```python
from build123d import *

# Parameters (mm, degrees)
IZIM2_W                     = 79
IZIM2_H                     = 44
IZIM2_R                     = 6.5
IZIM2_R_2                   = 1
IZIM2_R_3                   = 13
Y_KSEKLIK_EKSTR_ZYON1_DEPTH = 4
IZIM3_R                     = 15
IZIM3_R_2                   = 13
Y_KSEKLIK_EKSTR_ZYON2_DEPTH = 4


with BuildPart() as part:
    # Çizim2 → Yükseklik-Ekstrüzyon1 (new body)
    with BuildSketch(Plane(origin=(0, 0, 0), x_dir=(1, 0, 0), z_dir=(0, 1, 0))):
        with Locations((-17.5, 0)):
            Rectangle(IZIM2_W, IZIM2_H)
        with Locations(Location((0, 0, 0), (0, 0, 270))):
            Circle(IZIM2_R, mode=Mode.SUBTRACT)
        with Locations(Location((0, 12.5, 0), (0, 0, 270))):
            Circle(IZIM2_R_2, mode=Mode.SUBTRACT)
        with Locations(Location((0, -12.5, 0), (0, 0, 270))):
            Circle(IZIM2_R_2, mode=Mode.SUBTRACT)
        with Locations(Location((-35, 0, 0), (0, 0, 270))):
            Circle(IZIM2_R_3, mode=Mode.SUBTRACT)
    extrude(amount=Y_KSEKLIK_EKSTR_ZYON1_DEPTH)

    # Çizim3 → Yükseklik-Ekstrüzyon2 (add)
    with BuildSketch(Plane(origin=(0, 4, 0), x_dir=(1, 0, 0), z_dir=(0, 1, 0))):
        with Locations(Location((-35, 0, 0), (0, 0, 90))):
            Circle(IZIM3_R)
        with Locations(Location((-35, 0, 0), (0, 0, 270))):
            Circle(IZIM3_R_2, mode=Mode.SUBTRACT)
    extrude(amount=Y_KSEKLIK_EKSTR_ZYON2_DEPTH)


solid = part.part
```
Source: CAD feature listing. Evaluate the final solid. Frame: model axes, mm. A direction names the side the tool comes from. Coordinates: 2 decimals unless noted, no trailing zeros. Loops run counter-clockwise (first coordinate to the right, second up) from the corner with the lowest first, then second, coordinate; pieces in that order, holes last. Notation, with made-up numbers: (27.5, 25.5) -> (44.5, 25.5) arc R18 ccw to (44.5, 29.5) -> close; hole circle Ø5 at (54.25, 71.5). An arc over 180 degrees is marked (long way). One line per item, written item: value. Start each with the question number.
Q1. Section query B-B, the plane x = -35. Return the cut outline in (y, z).
Q2. Section query A-A, the plane x = 0. Return the cut outline in (y, z), and give its area (3 significant figures).
Q3. Line query: line 1 along X through (y, z) = (5, 0); line 2 along Y through (x, z) = (18, -5); line 3 along X through (y, z) = (5, -4.5). Output: solid intervals per line, ascending.
Q4. Section query C-C, the plane z = 0. Return the cut outline in (x, y), and give its area (3 significant figures).
Q5. Mould query, pull axis Z, two halves, no side actions, for faces 1 (the face through (-18, 2, -22)), 2 (the face through (-0.6, 2, -13.3)), 3 (the face through (-57, 2, 0)). Classes: pulls with the +Z half, pulls with the -Z half, needs draft (parallel to the pull), parting line crosses it, or undercut.
Q6. Set-up query: faces 4 (the face through (-22.11, 3.94, -1.69)), 5 (the face through (-47.65, 5.97, -8.06)). Return all of +Z, -Z, +X, -X, +Y, -Y with unobstructed straight access to the full face (end or side cutting, diameter ignored); none if empty.
Q7. Contact query for flat-ended pins moving along their axis: P1, Ø17, axis at x = 0, z = 0, coming from the +Y side; P2, Ø1.5, axis at y = 7, z = 6, coming from the +X side. Output: stop coordinate, or through.
Q8. Section query D-D, the plane y = 3. Return the cut outline in (x, z), and give its area (3 significant figures).
Results:
1. outline: (0, -22) -> (4, -22) -> (4, -15) -> (8, -15) -> (8, -13) -> (0, -13) -> close; (0, 13) -> (8, 13) -> (8, 15) -> (4, 15) -> (4, 22) -> (0, 22) -> close
2. outline: (0, -22) -> (4, -22) -> (4, -13.5) -> (0, -13.5) -> close; (0, -11.5) -> (4, -11.5) -> (4, -6.5) -> (0, -6.5) -> close; (0, 6.5) -> (4, 6.5) -> (4, 11.5) -> (0, 11.5) -> close; (0, 13.5) -> (4, 13.5) -> (4, 22) -> (0, 22) -> close
2. area: 108 mm^2
3. line 1: -50 to -48, -22 to -20
3. line 2: 0 to 4
3. line 3: -49.31 to -47.2, -22.8 to -20.69
4. outline: (-57, 0) -> (-48, 0) -> (-48, 8) -> (-50, 8) -> (-50, 4) -> (-57, 4) -> close; (-22, 0) -> (-6.5, 0) -> (-6.5, 4) -> (-20, 4) -> (-20, 8) -> (-22, 8) -> close; (6.5, 0) -> (22, 0) -> (22, 4) -> (6.5, 4) -> close
4. area: 176 mm^2
5. face 1: pulls with the -Z half
5. face 2: undercut
5. face 3: needs draft
6. face 4: +Y, -Y
6. face 5: +Y
7. P1: y = 4
7. P2: x = -20.95
8. outline: (-57, -22) -> (22, -22) -> (22, 22) -> (-57, 22) -> close; hole circle Ø26 at (-35, 0); hole circle Ø13 at (0, 0); hole circle Ø2 at (0, -12.5); hole circle Ø2 at (0, 12.5)
8. area: 2,810 mm^2
